Verification items for the finished model (mm, model axes). A direction names the side the tool comes from. Give positions to 0.01 mm unless a question says otherwise; leave off trailing zeros. One line per item, written item: value. Start each with the question number.
1. Access from +Z, -Z, +X, -X, +Y, -Y to the whole of each face (thin tool, end or side, straight path). Record for faces 1 (the flat face through (-88.9, -21, -2)), 2 (the cylindrical face through (-45.072, -93.287, 53.518)), 3 (the cylindrical face through (-1.24, 44.26, -77.48)), 4 (the flat face through (63.5, 221, 52)), 5 (the cylindrical face through (58.31, 92.99, 54.03)).
2. Mould release check, pull along Y, two halves, no side actions. Record for faces 6 (the flat face through (18.511, -86.049, -75.464)), 7 (the cylindrical face through (-45.07, 92.99, 54.03)), 8 (the cylindrical face through (76.38, -228.38, 10.05)), 9 (the flat face through (88.9, 117.5, -134.4)): pulls with the +Y half, pulls with the -Y half, needs draft (parallel to the pull), parting line crosses it, or undercut.
3. Gauge pin test, flat ends, axial feed: pin 1 (10 mm diameter, centred on x = 1, z = -121, fed in from +Y); pin 2 (12 mm diameter, centred on x = 58, y = 163, fed in from +Z); pin 3 (8 mm diameter, centred on x = 28.5, y = 135.5, fed in from -Z). Record the tip position at first contact, or that the pin passes through.
4. Sectioned sample at A-A (y = 58). Count the separate pieces of the cut face and the enclosed holes in it, plus the area to 3 significant figures.
5. Scan lines: L1, parallel to Y at x = 27.5, z = -80; L2, parallel to Z at x = 48, y = -41; L3, parallel to Z at x = -2, y = 51.5. Record each from-to range of solid material in increasing order. Write a range as [from, to].
from build123d import *

# Parameters (mm, degrees)
REVOLVE2_OUTLINE_W  = 25.39999999999995
REVOLVE2_OUTLINE_H  = 38.407758663
SKETCH3_R           = 107.54843304644665
SKETCH3_R_2         = 12.700000000000003
BOSS_EXTRUDE1_DEPTH = 177.79999999999998
BOSS_EXTRUDE2_START = -50.8
SKETCH4_R           = 107.54843304644665
BOSS_EXTRUDE2_DEPTH = 50.8
CUT_EXTRUDE1_START  = -508
CUT_EXTRUDE1_DEPTH  = 508
CIRPATTERN1_COUNT   = 6


# Read off the part's stored shape, not the designer's step: Revolve2
with BuildPart() as part:
    # Revolve2 outline → Revolve2 (revolve)
    with BuildSketch(Plane.YX):
        with BuildLine():
            add(Edge.make_bspline(
                [(12.7, 0), (65.56394076942757, 5.423140195743021), (107.548433046, 28.563700108)],
                knots=[0, 0, 0, 0.5115772122825497, 0.5115772122825497, 0.5115772122825497], degree=2))
            Line((12.7, 0), (107.548433046, 0))
            Line((107.548433046, 0), (107.548433046, 28.563700108))
        make_face()
        with BuildLine():
            add(Edge.make_bspline(
                [(107.548433046, 28.563700108), (124.74480096527253, 38.04180882229545), (140.116002229, 50.492241337)],
                knots=[0.5115772122825497, 0.5115772122825497, 0.5115772122825497, 0.7211133882490103, 0.7211133882490103, 0.7211133882490103], degree=2))
            Line((107.548433046, 28.563700108), (107.548433046, 0))
            add(Edge.make_bspline(
                [(177.8, 50.492241337), (174.25870908441857, 46.88747078495737), (156.1505738072, 29.8029081407884), (124.48137705008449, 8.138883125204057), (107.548433046, 0)],
                knots=[0.1400938920026617, 0.1400938920026617, 0.1400938920026617, 0.1875, 0.375, 0.5544007278163002, 0.5544007278163002, 0.5544007278163002], degree=2))
            Line((177.8, 50.492241337), (140.116002229, 50.492241337))
        make_face()
        with BuildLine():
            add(Edge.make_bspline(
                [(140.116002229, 50.492241337), (160.57462814001852, 67.06340821472577), (177.8, 88.9)],
                knots=[0.7211133882490103, 0.7211133882490103, 0.7211133882490103, 1, 1, 1], degree=2))
            Line((140.116002229, 50.492241337), (177.8, 50.492241337))
            Line((177.8, 50.492241337), (177.8, 88.9))
        make_face()
        Polygon((203.2, 50.492241337), (177.8, 50.492241337), (177.8, 0), (203.2, 0), (203.2, 40.64), align=None)
        with Locations((190.5, 69.6961206685)):
            Rectangle(REVOLVE2_OUTLINE_W, REVOLVE2_OUTLINE_H)
        Polygon((203.2, 0), (177.8, 0), (177.8, -88.9), (203.2, -88.9), (203.2, -40.64), align=None)
        with BuildLine():
            Line((205.432034985, 50.492241337), (203.2, 50.492241337))
            Line((203.2, 50.492241337), (203.2, 40.64))
            ThreePointArc((203.2, 40.64), (203.76499069, 45.690956334), (205.432034985, 50.492241337))
        make_face()
        with BuildLine():
            Line((203.2, 88.9), (203.2, 50.492241337))
            Line((203.2, 50.492241337), (205.432034985, 50.492241337))
            ThreePointArc((205.432034985, 50.492241337), (213.866613206, 59.976517745), (226.06, 63.5))
            Line((226.06, 63.5), (228.6, 63.5))
            Line((228.6, 63.5), (228.6, 88.9))
            Line((228.6, 88.9), (203.2, 88.9))
        make_face()
        with BuildLine():
            Line((203.2, -40.64), (203.2, -88.9))
            Line((203.2, -88.9), (228.6, -88.9))
            Line((228.6, -88.9), (228.6, -63.5))
            Line((228.6, -63.5), (226.06, -63.5))
            ThreePointArc((226.06, -63.5), (209.895538982, -56.804461018), (203.2, -40.64))
        make_face()
    revolve(axis=Axis((0, 0, 0), (1, 0, 0)))

    # Sketch3 → Boss-Extrude1 (add)
    with BuildSketch(Plane.ZY.offset(88.89999999999999)):
        Circle(SKETCH3_R)
        Circle(SKETCH3_R_2, mode=Mode.SUBTRACT)
    extrude(amount=-BOSS_EXTRUDE1_DEPTH)

    # Sketch4 → Boss-Extrude2 (add)
    with BuildSketch(Plane(origin=(88.89999999999999, 0, 0), x_dir=(0, 0, -1), z_dir=(1, 0, 0)).offset(BOSS_EXTRUDE2_START)):
        with Locations(Location((0, 0, 0), (0, 0, 180))):
            Circle(SKETCH4_R)
    extrude(amount=BOSS_EXTRUDE2_DEPTH)

    # Sketch5 → Cut-Extrude1 (cut)
    with BuildSketch(Plane(origin=(88.89999999999999, 0, 0), x_dir=(0, 0, -1), z_dir=(1, 0, 0)).offset(CUT_EXTRUDE1_START)):
        with BuildLine():
            Line((-28.680637108892512, 84.49362590578919), (-57.15, 168.36483451124818))
            ThreePointArc((-57.15, 168.36483451124818), (1.089e-14, 177.79999999999995), (57.15, 168.36483451124818))
            Line((57.15, 168.36483451124818), (28.680637108892512, 84.49362590578919))
            ThreePointArc((28.680637108892512, 84.49362590578919), (5.46e-15, 89.22864878322115), (-28.680637108892512, 84.49362590578919))
        make_face()
    cut_extrude1 = extrude(amount=CUT_EXTRUDE1_DEPTH, mode=Mode.SUBTRACT)

    # CirPattern1: Cut-Extrude1 ×6 about axis
    cirpattern1_axis = Axis((0, 2.4e-16, 1.8e-16), (1, 0, 0))
    for i in range(1, CIRPATTERN1_COUNT):
        add(cut_extrude1.rotate(cirpattern1_axis, i * 360 / CIRPATTERN1_COUNT), mode=Mode.SUBTRACT)


solid = part.part
Results are:
1. face 1: +Z, -Z, -X, +Y, -Y
1. face 2: -X
1. face 3: +X, -X
1. face 4: none
1. face 5: +X
2. face 6: undercut
2. face 7: undercut
2. face 8: parting line crosses it
2. face 9: needs draft
3. pin 1: stops at y = 166.84
3. pin 2: stops at z = 162.68
3. pin 3: stops at z = -154.91
4. separate pieces: 3
4. enclosed holes: 0
4. area: 36,700 mm^2
5. L1: y = [-186.79, -158.79], [-129.24, -91.22], [-39.52, 39.52], [91.22, 129.24], [158.79, 186.79]
5. L2: z = [-200.26, -173.01], [-79.25, 79.25], [173.01, 200.26]
5. L3: z = [-196.57, -170.18], [-72.87, 72.87], [170.18, 196.57]
